```python
from build123d import *

# Parameters (mm, degrees)
F2_DEPTH      = 12.5
F3_W          = 25
F3_H          = 7.5488379344
F4_DEPTH      = 12.5
F7_DEPTH      = 49.8707171405
F7_DEPTH_BACK = 0.7841883029
F8_DEPTH      = 7.5488379344
F11_DEPTH     = 25


with BuildPart() as f2:
    # F1 (on Right) → F2 (new body, symmetric)
    with BuildSketch(Plane.YZ):
        Polygon((-20, 0), (20, 0), (20, 7), (-20, 10.5), (-20, 7), align=None)
    extrude(amount=F2_DEPTH, both=True)


with BuildPart() as f4:
    # F3 (on face) → F4 (new body, symmetric)
    with BuildSketch(Plane(origin=(0, 0.7598077221, 8.6835168243), x_dir=(1, 0, 0), z_dir=(0, 0.0871669503, 0.9961937175))):
        with Locations((0, -24.6135462951)):
            Rectangle(F3_W, F3_H)
    extrude(amount=F4_DEPTH, both=True)


with BuildPart() as f7_tool:
    # F6 (on offset) → F7 (new body, two sides)
    with BuildSketch(Plane(origin=(0, 19.2373700353, -1.6832698781), x_dir=(-1, 0, 0), z_dir=(0, 0.9961937175, -0.0871669503))) as f7_sk:
        Polygon((-7, 5.7166950281), (7, 5.7166950281), (9, 5.7166950281), (7, 8.7166950281), (-7, 8.7166950281), (-9, 5.7166950281), align=None)
    extrude(amount=-F7_DEPTH)
    extrude(f7_sk.sketch, amount=F7_DEPTH_BACK)


with BuildPart() as f2_1:
    add(f2.part)

    # F7: cut by f7_tool
    add(f7_tool.part, mode=Mode.SUBTRACT)

    # F10 (on face) → F11 (cut, through all)
    with BuildSketch(Plane.YZ.offset(12.5)):
        Polygon((-19.9651202156, 0), (-19.0536159684, 10.4171913972), (-20, 10.5), (-20, 0), align=None)
        Polygon((20, 0), (20, 7), (19.3875, 0), align=None)
    extrude(amount=-F11_DEPTH, mode=Mode.SUBTRACT)


with BuildPart() as f4_1:
    add(f4.part)

    # F7: cut by f7_tool
    add(f7_tool.part, mode=Mode.SUBTRACT)

    # F8 (cut, through all): a face of the model
    f8_faces = [f4_1.faces().sort_by_distance(p)[0] for p in [
        (0, -27.5087747318, 11.2874970991),
    ]]
    extrude(f8_faces, amount=-F8_DEPTH, mode=Mode.SUBTRACT)


solid = f2_1.part
```
For this review, take the finished solid that the model builds, in its own axes (mm). A direction names the side the tool comes from. Round coordinates to 2 decimals unless told otherwise and drop trailing zeros. Order: outer loops, then holes, each group sorted by start corner. A loop starts at its lowest first (then second) coordinate and runs counter-clockwise, first axis right, second up.
Q1. Insertion check: P1, Ø6, axis at x = 10, z = 5.5, coming from the -Y side. The pin has a flat end and moves straight along its axis. Give the tip position at first contact, or say it passes through.
Findings below:
P1: stops at y = -19.75
Q2. Wall thickness on line 1 (X direction, y = -7, z = 8); line 2 (Z direction, x = 7.75, y = 8.5); line 3 (Z direction, x = 7.5, y = -1): over which ranges is each line inside the solid? List them lowest first.
Findings below:
line 1: x = -12.5 to -7.9, 7.9 to 12.5
line 2: z = 0 to 4.99, 6.88 to 8.01
line 3: z = 0 to 5.83, 8.08 to 8.84
Q3. We need section D-D, the plane x = 10. Give the boundary of the cut face in (y, z).
Findings below:
outline: (-19.97, 0) - (19.39, 0) - (20, 7) - (-19.05, 10.42) - close
Q4. We need section C-C, the plane y = 7.5. Give the boundary of the cut face in (x, z).
Findings below:
outline: (-12.5, 0) - (12.5, 0) - (12.5, 8.09) - (7, 8.09) - (9, 5.08) - (-9, 5.08) - (-7, 8.09) - (-12.5, 8.09) - close
Q5. We need section A-A, the plane z = 8. Give the boundary of the cut face in (x, y), plus the area to 3 significant figures.
Findings below:
outline: (-12.5, -19.27) - (-8.62, -19.27) - (-7, 8.57) - (-12.5, 8.57) - close; (7, 8.57) - (8.62, -19.27) - (12.5, -19.27) - (12.5, 8.57) - close
area: 261 mm2
Q6. Machinability: for faces 1 (the flat face through (9.788, 0.747, 8.685)), 2 (the flat face through (-8.01, 0.07, 7.22)), which of the approach directions +Z, -Z, +X, -X, +Y, -Y give a long, thin tool a straight path to every point of the face, cutting with its end or side? Answer none if there is none.
Findings below:
face 1: +Z, +X, -X, +Y
face 2: none
Q7. We need section B-B, the plane x = -8.5. Give the boundary of the cut face in (y, z).
Findings below:
outline: (-19.97, 0) - (19.39, 0) - (19.74, 4.01) - (-19.32, 7.43) - close; (-19.25, 8.18) - (19.8, 4.76) - (20, 7) - (-19.05, 10.42) - close
Q8. Mouldability with a two-part tool opening along X and no side actions: class faces 3 (the flat face through (0.126, -0.062, 5.744)), 4 (the flat face through (12.5, 0, 4)), 5 (the flat face through (0.175, -19.617, 3.978)), 6 (the flat face through (7.986, 0.071, 7.259)) as pulls with the +X half, pulls with the -X half, needs draft (parallel to the pull), parting line crosses it, or undercut.
Findings below:
face 3: undercut
face 4: pulls with the +X half
face 5: needs draft
face 6: undercut
